Can you work these out from the model? Positions are in its coordinate system, mm. A direction names the side the tool comes from. Give positions to 0.01 mm unless a question says otherwise; leave off trailing zeros. Loops run counter-clockwise (first coordinate to the right, second up) from the corner with the lowest first, then second, coordinate; pieces in that order, holes last. Notation, with made-up numbers: M 16,4.25 L 21,4.25 A17 ccw 21,23.25 Z; hole C 8,56.5 d2. An arc over 180 degrees is marked long. One line per item, written item: value. Start each with the question number.
from build123d import *

# Parameters (mm, degrees)
SKETCH1_R           = 73.025
BOSS_EXTRUDE1_DEPTH = 6.35
SKETCH2_R           = 73.025
SKETCH2_R_2         = 66.548
BOSS_EXTRUDE2_DEPTH = 25.4
CUT_EXTRUDE1_REACH  = 110.043
SKETCH3_R           = 19.304


with BuildPart() as part:
    # Sketch1 → Boss-Extrude1 (new body)
    with BuildSketch(Plane(origin=(0, 0, 0), x_dir=(1, 0, 0), z_dir=(0, 1, 0))):
        with Locations(Location((0, 0, 0), (0, 0, 270))):
            Circle(SKETCH1_R)
    extrude(amount=BOSS_EXTRUDE1_DEPTH)

    # Sketch2 → Boss-Extrude2 (add)
    with BuildSketch(Plane(origin=(0, 6.35, 0), x_dir=(1, 0, 0), z_dir=(0, 1, 0))):
        with Locations(Location((0, 0, 0), (0, 0, 270))):
            Circle(SKETCH2_R)
        with Locations(Location((0, 0, 0), (0, 0, 270))):
            Circle(SKETCH2_R_2, mode=Mode.SUBTRACT)
    extrude(amount=BOSS_EXTRUDE2_DEPTH)

    # Sketch3 → Cut-Extrude1 (cut, up to next)
    with BuildSketch(Plane.XZ, mode=Mode.PRIVATE) as cut_extrude1_sk1:
        with Locations(Location((0, 0, 0), (0, 0, 270))):
            Circle(SKETCH3_R)
    cut_extrude1_tool1 = extrude(cut_extrude1_sk1.sketch, amount=-CUT_EXTRUDE1_REACH, mode=Mode.PRIVATE) & part.part
    add(cut_extrude1_tool1.solids().sort_by_distance((0, 0, 0))[0], mode=Mode.SUBTRACT)


solid = part.part
Q1. Which directions (+Z, -Z, +X, -X, +Y, -Y) give clear straight access to the entire face, cutting with the end or side of a thin tool? Please do faces 4 (the face through (65.982, 18.872, -8.663)), 5 (the face through (-11.746, 3.131, 15.319)).
Q2. If we section it at A-A, the plane z = 0: Write out the boundary of the cut face in (x, y) (3 decimals).
Q3. For P1, Ø1.5, axis at x = -34.5, z = -50, coming from the +Y side; P2, Ø8, axis at x = 41.5, y = 23.5, coming from the -Z side; P3, Ø12, axis at x = -54.5, y = 24, coming from the -Z side, each with a flat end and sliding along its axis, tell me the tip position at first contact or that it passes through.
Q4. I need wall thicknesses on line 1 along X through (y, z) = (17, 0) (3 decimals); line 2 along X through (y, z) = (4, 0) (3 decimals); line 3 along Y through (x, z) = (-30.5, -55.5). Which ranges of each line are inside material? Lowest first, please.
Q5. If we section it at D-D, the plane z = 52: Write out the boundary of the cut face in (x, y).
Q6. If we section it at C-C, the plane y = 12.5: Write out the boundary of the cut face in (x, z) (3 decimals), plus the area to 3 significant figures.
Q7. If we mould it in two halves opening along X, with no side actions, what happens to faces 1 (the face through (-14, 6.35, 14)), 2 (the face through (-65, 31.75, -17)), 3 (the face through (21.935, 15.653, 69.653))? For each: released by +X, released by -X, zero draft, split by the parting line, or undercut.
Q8. If we section it at B-B, the plane x = 0: Write out the boundary of the cut face in (y, z) (3 decimals).
Response:
1. face 4: +Y
1. face 5: +Y, -Y
2. outline: M -73.025,0 L -19.304,0 L -19.304,6.35 L -66.548,6.35 L -66.548,31.75 L -73.025,31.75 Z; M 19.304,0 L 73.025,0 L 73.025,31.75 L 66.548,31.75 L 66.548,6.35 L 19.304,6.35 Z
3. P1: y = 6.35
3. P2: z = -62.66
3. P3: z = -54.59
4. line 1: -73.025 to -66.548, 66.548 to 73.025
4. line 2: -73.025 to -19.304, 19.304 to 73.025
4. line 3: 0 to 6.35
5. outline: M -51.27,0 L 51.27,0 L 51.27,31.75 L 41.53,31.75 L 41.53,6.35 L -41.53,6.35 L -41.53,31.75 L -51.27,31.75 Z
6. outline: C 0,0 d146.05; hole C 0,0 d133.096
6. area: 2,840 mm^2
7. face 1: undercut
7. face 2: zero draft
7. face 3: split by the parting line
8. outline: M 0,-73.025 L 31.75,-73.025 L 31.75,-66.548 L 6.35,-66.548 L 6.35,-19.304 L 0,-19.304 Z; M 0,19.304 L 6.35,19.304 L 6.35,66.548 L 31.75,66.548 L 31.75,73.025 L 0,73.025 Z
